from build123d import *

# Parameters (mm, degrees)
F1_DEPTH = 13
F2_W     = 110
F2_H     = 20
F3_DEPTH = 25
F4_W     = 110
F4_H     = 20
F5_DEPTH = 25


with BuildPart() as f1:
    # F0 (on Front) → F1 (new body)
    with BuildSketch(Plane.XZ):
        with BuildLine():
            Line((218.799954, 176.439716), (-38.200046, 176.439716))
            ThreePointArc((-38.200046, 176.439716), (-52.342182, 170.581852), (-58.200046, 156.439716))
            Line((-58.200046, 156.439716), (-58.200046, -13.560284))
            ThreePointArc((-58.200046, -13.560284), (-52.342182, -27.70242), (-38.200046, -33.560284))
            Line((-38.200046, -33.560284), (218.799954, -33.560284))
            ThreePointArc((218.799954, -33.560284), (232.942089, -27.70242), (238.799954, -13.560284))
            Line((238.799954, -13.560284), (238.799954, 156.439716))
            ThreePointArc((238.799954, 156.439716), (232.942089, 170.581852), (218.799954, 176.439716))
        make_face()
    extrude(amount=F1_DEPTH)

    # F2 (on face) → F3 (cut)
    with BuildSketch(Plane.XZ.offset(13)):
        with Locations((-9.645737, 134.683969)):
            Rectangle(F2_W, F2_H)
    extrude(amount=-F3_DEPTH, mode=Mode.SUBTRACT)

    # F4 (on face) → F5 (cut)
    with BuildSketch(Plane.XZ.offset(13)):
        with Locations((-10.065921, 96.247018)):
            Rectangle(F4_W, F4_H)
    extrude(amount=-F5_DEPTH, mode=Mode.SUBTRACT)


solid = f1.part
Verification items for the finished model (mm, model axes). A direction names the side the tool comes from. Give positions to 0.01 mm unless a question says otherwise; leave off trailing zeros. Write each loop counter-clockwise with the first axis right and the second up, starting at its lowest first coordinate (ties: lowest second). Pieces come first, ordered by that corner, then holes. Notation, with made-up numbers: M 54,65 L 92,65 A22 ccw 92,75 Z; hole C 18,46.25 d6. An arc over 180 degrees is marked long. Use CSV: the item, a comma, the result in double quotes.
1) Access from +Z, -Z, +X, -X, +Y, -Y to the whole of each face (thin tool, end or side, straight path). Record for faces 1 (the face through (238.8, -6, 70)), 2 (the face through (-7, -7, 144.684)).
Final values:
face 1,"+Z, -Z, +X, +Y, -Y"
face 2,"-X, +Y, -Y"
2) Material ranges on line 1 along Z through (x, y) = (36, -10.5); line 2 along X through (y, z) = (-1, 89); line 3 along X through (y, z) = (-6.25, 134), recorded low to high.
Final values:
line 1,"-33.56 to 86.25, 106.25 to 124.68, 144.68 to 176.44"
line 2,"44.93 to 238.8"
line 3,"45.35 to 238.8"
3) Cross-section at B-B (y = -10). Enter the section's corners in (x, z).
Final values:
outline,"M -58.2,-13.56 A20 ccw -38.2,-33.56 L 218.8,-33.56 A20 ccw 238.8,-13.56 L 238.8,156.44 A20 ccw 218.8,176.44 L -38.2,176.44 A20 ccw -58.2,156.44 L -58.2,144.68 L 45.35,144.68 L 45.35,124.68 L -58.2,124.68 L -58.2,106.25 L 44.93,106.25 L 44.93,86.25 L -58.2,86.25 Z"
4) Go/stop test with a flat-tipped pin: pin 1 Ø4 at (y, z) = (-8, 139) entering from -X. Record where the tip stops, or that it passes through.
Final values:
pin 1,"x = 45.35"
5) Release check for a two-part mould opening along Z. For faces 3 (the face through (-7, -7, 124.684)), 4 (the face through (-58.2, -6, 116)), 5 (the face through (89, -6, -33.56)) record: released by +Z, released by -Z, zero draft, split by the parting line, or undercut.
Final values:
face 3,"undercut"
face 4,"zero draft"
face 5,"released by -Z"
6) Cross-section at C-C (z = 103). Enter the section's corners in (x, y).
Final values:
outline,"M 44.93,-13 L 238.8,-13 L 238.8,0 L 44.93,0 Z"
7) Cross-section at A-A (x = -22.5). Enter the section's corners in (y, z).
Final values:
outline,"M -13,-33.56 L 0,-33.56 L 0,86.25 L -13,86.25 Z; M -13,106.25 L 0,106.25 L 0,124.68 L -13,124.68 Z; M -13,144.68 L 0,144.68 L 0,176.44 L -13,176.44 Z"
